Here's how the part is built. I have some questions about the finished solid (model axes, mm). Coordinates: 2 decimals unless noted, no trailing zeros. Loops run counter-clockwise (first coordinate to the right, second up) from the corner with the lowest first, then second, coordinate; pieces in that order, holes last. Notation, with made-up numbers: (14.25, -21.75) - (60.25, -21.75) arc R18 cw to (60.25, -2.75) - close; hole circle Ø2 at (60.5, -0.75). An arc over 180 degrees is marked (long way). Use a Markdown table: item, result.
```python
from build123d import *

# Parameters (mm, degrees)
SKETCH1_W                      = 50
SKETCH1_H                      = 65
BOSS_EXTRUDE1_DEPTH            = 5
CBORE_START                    = 2
CBORE_FOR_M3_SHCS1_OUTLINE_R   = 3.25
CBORE_FOR_M3_SHCS1_DEPTH       = 3
CBORE_FOR_M3_SHCS1_2_OUTLINE_R = 1.8
CBORE_FOR_M3_SHCS1_2_DEPTH     = 2
SKETCH5_W                      = 66
SKETCH5_H                      = 8
BOSS_EXTRUDE2_DEPTH            = 5
FILLET1_R                      = 3
M3_CLEARANCE_HOLE1_D           = 3.6


# Read off the part's stored shape, not the designer's step: CBORE for M3 SHCS1
with BuildPart() as part:
    # Sketch1 → Boss-Extrude1 (new body)
    with BuildSketch(Plane(origin=(0, 0, 0), x_dir=(1, 0, 0), z_dir=(0, 1, 0))):
        Rectangle(SKETCH1_W, SKETCH1_H)
    extrude(amount=BOSS_EXTRUDE1_DEPTH)

    # CBORE for M3 SHCS1 outline → CBORE for M3 SHCS1 (cut)
    with BuildSketch(Plane(origin=(0, 0, 0), x_dir=(1, 0, 0), z_dir=(0, 1, 0)).offset(CBORE_START)):
        with Locations((19.75, -26.5)):
            Circle(CBORE_FOR_M3_SHCS1_OUTLINE_R)
        with Locations((-19.75, 26.5)):
            Circle(CBORE_FOR_M3_SHCS1_OUTLINE_R)
        with Locations((-19.75, -26.5)):
            Circle(CBORE_FOR_M3_SHCS1_OUTLINE_R)
        with Locations((19.75, 26.5)):
            Circle(CBORE_FOR_M3_SHCS1_OUTLINE_R)
    extrude(amount=CBORE_FOR_M3_SHCS1_DEPTH, mode=Mode.SUBTRACT)

    # CBORE for M3 SHCS1 2 outline → CBORE for M3 SHCS1 2 (cut)
    with BuildSketch(Plane(origin=(0, 0, 0), x_dir=(1, 0, 0), z_dir=(0, 1, 0))):
        with Locations((19.75, -26.5)):
            Circle(CBORE_FOR_M3_SHCS1_2_OUTLINE_R)
        with Locations((-19.75, 26.5)):
            Circle(CBORE_FOR_M3_SHCS1_2_OUTLINE_R)
        with Locations((-19.75, -26.5)):
            Circle(CBORE_FOR_M3_SHCS1_2_OUTLINE_R)
        with Locations((19.75, 26.5)):
            Circle(CBORE_FOR_M3_SHCS1_2_OUTLINE_R)
    extrude(amount=CBORE_FOR_M3_SHCS1_2_DEPTH, mode=Mode.SUBTRACT)

    # Sketch5 → Boss-Extrude2 (add)
    with BuildSketch(Plane(origin=(0, 5, 0), x_dir=(1, 0, 0), z_dir=(0, 1, 0))):
        Rectangle(SKETCH5_W, SKETCH5_H)
    extrude(amount=-BOSS_EXTRUDE2_DEPTH)

    # Fillet1
    fillet1_edges = [part.edges().sort_by_distance(p)[0] for p in [
        (33, 2.5, 4),
        (-33, 2.5, -4),
        (33, 2.5, -4),
        (25, 2.5, 4),
        (-25, 2.5, 4),
        (-33, 2.5, 4),
        (25, 2.5, -4),
        (-25, 2.5, -4),
        (25, 2.5, 32.5),
        (-25, 2.5, 32.5),
        (-25, 2.5, -32.5),
        (25, 2.5, -32.5),
    ]]
    fillet(fillet1_edges, radius=FILLET1_R)

    # M3 Clearance Hole1 (through all)
    with Locations(Plane(origin=(0, 5, 0), x_dir=(1, 0, 0), z_dir=(0, 1, 0))):
        with Locations((-29, 0), (29, 0)):
            Hole(M3_CLEARANCE_HOLE1_D / 2)


solid = part.part
```
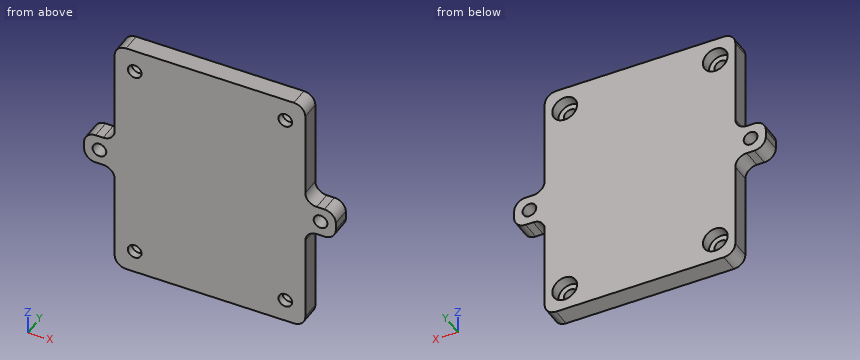
Q1. I want a section at D-D, the plane y = 1.2. Give the number of separate pieces and of enclosed holes in the cut face, then the cut area to 3 significant figures.
Check values:
| item | result |
|---|---|
| separate pieces | 1 |
| enclosed holes | 6 |
| area | 3,310 mm^2 |
Q2. Please list where these lines run through material, in increasing order: L1, parallel to Z at x = 19.75, y = 0.65; L2, parallel to X at y = 3.25, z = 26.5; L3, parallel to X at y = 1.4, z = -26.5. Write a range as from..to.
Check values:
| item | result |
|---|---|
| L1 | -32.5..-28.3, -24.7..24.7, 28.3..32.5 |
| L2 | -25..-23, -16.5..16.5, 23..25 |
| L3 | -25..-21.55, -17.95..17.95, 21.55..25 |
Q3. I want a section at A-A, the plane z = 0. Write out the boundary of the cut face in (x, y).
Check values:
| item | result |
|---|---|
| outline | (-33, 0) - (-30.8, 0) - (-30.8, 5) - (-33, 5) - close; (-27.2, 0) - (27.2, 0) - (27.2, 5) - (-27.2, 5) - close; (30.8, 0) - (33, 0) - (33, 5) - (30.8, 5) - close |
Q4. Will these pins go through, and if not, where does the flat tip stop? P1, Ø8.5, axis at x = 19.75, z = -26.5, coming from the +Y side; P2, Ø5, axis at x = -19.75, z = 26.5, coming from the +Y side; P3, Ø2, axis at x = -29, y = 2, coming from the +Z side; P4, Ø1.5, axis at y = 2, z = -22.5, coming from the +X side.
Check values:
| item | result |
|---|---|
| P1 | y = 5 |
| P2 | y = 2 |
| P3 | z = 4 |
| P4 | x = 25 |
Q5. I want a section at B-B, the plane x = -19.75. Write out the boundary of the cut face in (y, z).
Check values:
| item | result |
|---|---|
| outline | (0, -32.5) - (5, -32.5) - (5, -29.75) - (2, -29.75) - (2, -28.3) - (0, -28.3) - close; (0, -24.7) - (2, -24.7) - (2, -23.25) - (5, -23.25) - (5, 23.25) - (2, 23.25) - (2, 24.7) - (0, 24.7) - close; (0, 28.3) - (2, 28.3) - (2, 29.75) - (5, 29.75) - (5, 32.5) - (0, 32.5) - close |
Q6. I want a section at C-C, the plane x = 29. Write out the boundary of the cut face in (y, z), then the cut area to 3 significant figures.
Check values:
| item | result |
|---|---|
| outline | (0, -4) - (5, -4) - (5, -1.8) - (0, -1.8) - close; (0, 1.8) - (5, 1.8) - (5, 4) - (0, 4) - close |
| area | 22.0 mm^2 |
